```python
from build123d import *

# Parameters (mm, degrees)
SKETCH001_R     = 6
PAD_DEPTH       = 3.1
SKETCH_R        = 4.05
POCKET_DEPTH    = 3.101
SKETCH002_R     = 4.5
POCKET001_DEPTH = 1


with BuildPart() as part:
    # Sketch001 → Pad (new body)
    with BuildSketch(Plane.XY):
        Circle(SKETCH001_R)
    extrude(amount=PAD_DEPTH)

    # Sketch → Pocket (cut, through all)
    with BuildSketch(Plane.XY):
        Circle(SKETCH_R)
    extrude(amount=POCKET_DEPTH, mode=Mode.SUBTRACT)

    # Sketch002 → Pocket001 (cut)
    with BuildSketch(Plane.XY):
        Circle(SKETCH002_R)
    extrude(amount=POCKET001_DEPTH, mode=Mode.SUBTRACT)


solid = part.part
```
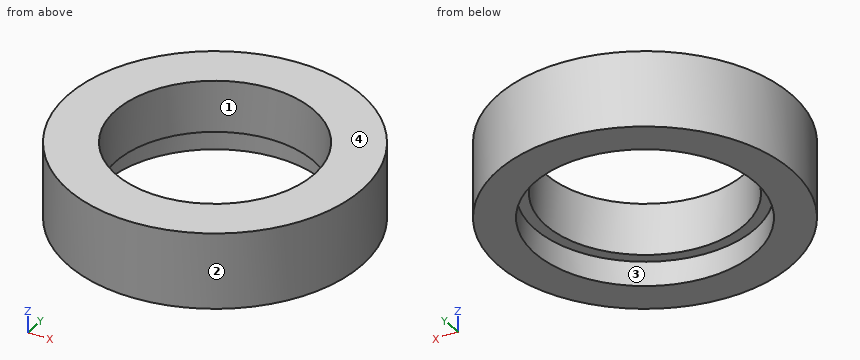
The listing builds one solid part. Answer for the finished solid, in the listing's coordinates (mm). Face numbers are marked on the shaded views. Round coordinates to 2 decimals unless told otherwise and drop trailing zeros. Loops run counter-clockwise (first coordinate to the right, second up) from the corner with the lowest first, then second, coordinate; pieces in that order, holes last.
Q1. Given pin 1 Ø1 at (y, z) = (-3.5, 1.5) entering from +X; pin 2 Ø1 at (x, z) = (-1, 0.5) entering from +Y; pin 3 Ø2.5 at (x, y) = (1.5, 1.5) entering from -Z; pin 4 Ø1.5 at (x, z) = (-3, 2) entering from +Y, each flat-ended and moving along its own axis, determine where each tip first touches the part or whether it passes through.
Q2. Section A-A, the plane y = 0 is taken. Determine the outline of the cut face in (x, z), then the cut area to 3 significant figures.
Q3. Section D-D, the plane y = 4.25 is taken. Determine the outline of the cut face in (x, z).
Q4. For a pull along Y with two mould halves and no side action, classify the marked faces 1, 2, 3 and 4 as released by +Y, released by -Y, zero draft, split by the parting line, or undercut.
Q5. Section C-C, the plane z = 0.3 is taken. Determine the outline of the cut face in (x, y).
Q6. Find the intervals of material crossed by line 1 (Y direction, x = 0, z = 0.5); line 2 (Y direction, x = 0, z = 2.45); line 3 (X direction, y = 2.5, z = 0.4), in increasing order.
Completed:
1. pin 1: stops at x = 5.2
1. pin 2: stops at y = 5.98
1. pin 3: passes through
1. pin 4: stops at y = 5.56
2. outline: (-6, 0) - (-4.5, 0) - (-4.5, 1) - (-4.05, 1) - (-4.05, 3.1) - (-6, 3.1) - close; (4.05, 1) - (4.5, 1) - (4.5, 0) - (6, 0) - (6, 3.1) - (4.05, 3.1) - close
2. area: 11.2 mm2
3. outline: (-4.24, 0) - (-1.48, 0) - (-1.48, 1) - (1.48, 1) - (1.48, 0) - (4.24, 0) - (4.24, 3.1) - (-4.24, 3.1) - close
4. face 1: undercut
4. face 2: split by the parting line
4. face 3: undercut
4. face 4: zero draft
5. outline: circle Ø12 at (0, 0); hole circle Ø9 at (0, 0)
6. line 1: y = -6 to -4.5, 4.5 to 6
6. line 2: y = -6 to -4.05, 4.05 to 6
6. line 3: x = -5.45 to -3.74, 3.74 to 5.45
